from build123d import *

# Parameters (mm, degrees)
SCHIZZO1_R                   = 12.5
SCHIZZO1_R_2                 = 9.5
ESTRUSIONE_ESTRUSIONE1_DEPTH = 13.5
SCHIZZO2_W                   = 9
SCHIZZO2_H                   = 12
TAGLIO_ESTRUSIONE1_DEPTH     = 23.24297642
ESTRUSIONE_ESTRUSIONE2_DEPTH = 5
SCHIZZO3_R                   = 75.5
SCHIZZO3_R_2                 = 67.5
BOSS_EXTRUDE1_DEPTH          = 3
SKETCH1_W                    = 3
SKETCH1_H                    = 7.5
SKETCH2_R                    = 72.5
SKETCH2_R_2                  = 70.5
CUT_EXTRUDE1_DEPTH           = 3


with BuildPart() as part:
    # Schizzo1 → Estrusione-Estrusione1 (new body)
    with BuildSketch(Plane(origin=(0, 0, 0), x_dir=(1, 0, 0), z_dir=(0, 1, 0))):
        with Locations(Location((0, 0, 0), (0, 0, 270))):
            Circle(SCHIZZO1_R)
        with Locations(Location((0, 0, 0), (0, 0, 270))):
            Circle(SCHIZZO1_R_2, mode=Mode.SUBTRACT)
    extrude(amount=ESTRUSIONE_ESTRUSIONE1_DEPTH)

    # Schizzo2 → Taglio-Estrusione1 (cut, through all)
    with BuildSketch(Plane(origin=(0, 13.5, 0), x_dir=(1, 0, 0), z_dir=(0, 1, 0))):
        with Locations((-11.865459931, 0)):
            Rectangle(SCHIZZO2_W, SCHIZZO2_H)
    extrude(amount=-TAGLIO_ESTRUSIONE1_DEPTH, mode=Mode.SUBTRACT)

    # Schizzo5 → Estrusione-Estrusione2 (add, symmetric)
    with BuildSketch(Plane(origin=(0, 0, 0), x_dir=(0, 0, -1), z_dir=(1, 0, 0))):
        with BuildLine():
            Line((-64.5, 26), (-64.5, 33.5))
            ThreePointArc((-64.5, 33.5), (-37.371539554, 26.433997159), (-12.5, 13.5))
            Line((-12.5, 13.5), (-11.5, 13.5))
            Line((-11.5, 13.5), (-11.5, 0))
            Line((-11.5, 0), (-12.5, 0))
            ThreePointArc((-12.5, 0), (-43.534901683, 17.988326497), (-78.5, 26))
            Line((-78.5, 26), (-64.5, 26))
        make_face()
    estrusione_estrusione2 = extrude(amount=ESTRUSIONE_ESTRUSIONE2_DEPTH, both=True)

    # Schizzo3 → Boss-Extrude1 (add)
    with BuildSketch(Plane(origin=(0, 26, 0), x_dir=(1, 0, 0), z_dir=(0, 1, 0))):
        with Locations(Location((0, 0, 0), (0, 0, 266.202798448))):
            Circle(SCHIZZO3_R)
        with Locations(Location((0, 0, 0), (0, 0, 265.751977333))):
            Circle(SCHIZZO3_R_2, mode=Mode.SUBTRACT)
    extrude(amount=BOSS_EXTRUDE1_DEPTH)

    # Sketch1 → Revolve1 (revolve)
    with BuildSketch(Plane(origin=(0, 0, 0), x_dir=(0, 0, -1), z_dir=(1, 0, 0)), mode=Mode.PRIVATE) as revolve1_sk:
        with Locations((77, 29.75)):
            Rectangle(SKETCH1_W, SKETCH1_H)
        with Locations((66, 29.75)):
            Rectangle(SKETCH1_W, SKETCH1_H)
    revolve(revolve1_sk.sketch.rotate(Axis((0, 39.375, 0), (0, -1, 0)), 180), axis=Axis((0, 39.375, 0), (0, -1, 0)))

    # Mirror1: Estrusione-Estrusione2 across plane
    add(estrusione_estrusione2.mirror(Plane.XY))

    # Sketch2 → Cut-Extrude1 (cut)
    with BuildSketch(Plane(origin=(0, 29, 0), x_dir=(1, 0, 0), z_dir=(0, 1, 0))):
        with Locations(Location((0, 0, 0), (0, 0, 270))):
            Circle(SKETCH2_R)
        with Locations(Location((0, 0, 0), (0, 0, 270))):
            Circle(SKETCH2_R_2, mode=Mode.SUBTRACT)
    extrude(amount=-CUT_EXTRUDE1_DEPTH, mode=Mode.SUBTRACT)


solid = part.part
For this review, take the finished solid that the model builds, in its own axes (mm). A direction names the side the tool comes from. Round coordinates to 2 decimals unless told otherwise and drop trailing zeros. Loops run counter-clockwise (first coordinate to the right, second up) from the corner with the lowest first, then second, coordinate; pieces in that order, holes last. Notation, with made-up numbers: (74, -22.75) - (118, -22.75) arc R24 ccw to (118, 4.25) - close; hole circle Ø10 at (47.5, 17.25). An arc over 180 degrees is marked (long way). One line per question, with ' | ' between items.
Q1. For line 1 along X through (y, z) = (30, 0); line 2 along X through (y, z) = (27.4, 0); line 3 along Z through (x, y) = (41.5, 30), list the stretches that pass through material, from the lowest coordinate up. Write a range as [from, to].
Taken from the geometry:
line 1: x = [-78.5, -75.5], [-67.5, -64.5], [64.5, 67.5], [75.5, 78.5] | line 2: x = [-78.5, -72.5], [-70.5, -64.5], [64.5, 70.5], [72.5, 78.5] | line 3: z = [-66.63, -63.07], [-53.24, -49.38], [49.38, 53.24], [63.07, 66.63]
Q2. Take a section at B-B (y = 23). Give the boundary of the cut face in (x, z).
Taken from the geometry:
outline: (-5, -59.41) - (5, -59.41) - (5, -29.3) - (-5, -29.3) - close; (-5, 29.3) - (5, 29.3) - (5, 59.41) - (-5, 59.41) - close
Q3. Take a section at D-D (x = -46.5). Give the boundary of the cut face in (y, z), and give its area (3 significant figures).
Taken from the geometry:
outline: (26, -63.25) - (33.5, -63.25) - (33.5, -59.48) - (29, -59.48) - (29, -55.62) - (26, -55.62) - close; (26, -52.99) - (29, -52.99) - (29, -48.93) - (33.5, -48.93) - (33.5, -44.7) - (26, -44.7) - close; (26, 44.7) - (33.5, 44.7) - (33.5, 48.93) - (29, 48.93) - (29, 52.99) - (26, 52.99) - close; (26, 55.62) - (29, 55.62) - (29, 59.48) - (33.5, 59.48) - (33.5, 63.25) - (26, 63.25) - close | area: 167 mm²
Q4. Tool access review of faces 1 (the cylindrical face through (-20.28, 31.28, 64.38)), 2 (the flat face through (-9, 7, -6)), 3 (the flat face through (35, 33.5, -55)), 4 (the flat face through (67, 26, 0)): name each direction out of +Z, -Z, +X, -X, +Y, -Y from which nothing blocks a thin tool from reaching the whole face with its end or side.
Taken from the geometry:
face 1: +Y | face 2: -X, +Y, -Y | face 3: +Z, -Z, +X, -X, +Y | face 4: +Z, -Z, +X, -Y
Q5. Take a section at A-A (z = 0). Give the boundary of the cut face in (x, y).
Taken from the geometry:
outline: (-78.5, 26) - (-72.5, 26) - (-72.5, 29) - (-75.5, 29) - (-75.5, 33.5) - (-78.5, 33.5) - close; (-70.5, 26) - (-64.5, 26) - (-64.5, 33.5) - (-67.5, 33.5) - (-67.5, 29) - (-70.5, 29) - close; (9.5, 0) - (12.5, 0) - (12.5, 13.5) - (9.5, 13.5) - close; (64.5, 26) - (70.5, 26) - (70.5, 29) - (67.5, 29) - (67.5, 33.5) - (64.5, 33.5) - close; (72.5, 26) - (78.5, 26) - (78.5, 33.5) - (75.5, 33.5) - (75.5, 29) - (72.5, 29) - close
Q6. For pin 1 (1 mm diameter, centred on y = 29.5, z = -52, fed in from +X); pin 2 (1.7 mm diameter, centred on x = 1, z = -71.5, fed in from +Y); pin 3 (2 mm diameter, centred on x = 12.5, z = 8.5, fed in from -Y); pin 4 (3 mm diameter, centred on y = 9.5, z = -23.5, fed in from -X), all flat-tipped, find the tip position at first contact; note any pin that passes through.
Taken from the geometry:
pin 1: stops at x = 59.25 | pin 2: stops at y = 26 | pin 3: passes through | pin 4: stops at x = -5
Q7. The part is to be moulded in two halves that separate along X. For faces 5 (the flat face through (-5, 18, 37)), 6 (the cylindrical face through (-23.579, 29.803, 74.875)), 7 (the flat face through (5, 18, -37)), 8 (the flat face through (-72, 26, 12)), say which applies: released by +X, released by -X, zero draft, split by the parting line, or undercut.
Taken from the geometry:
face 5: undercut | face 6: split by the parting line | face 7: undercut | face 8: zero draft
